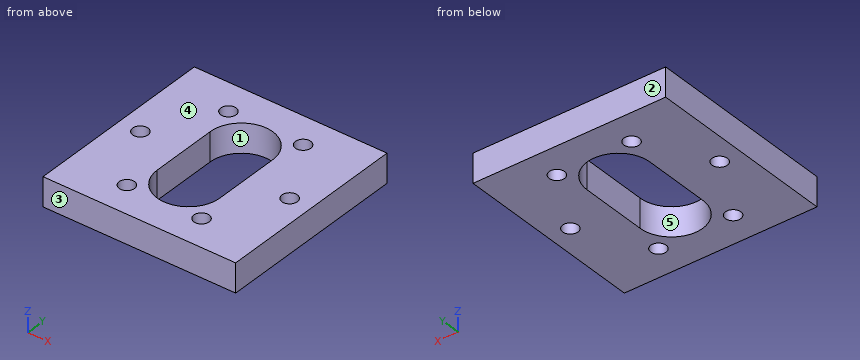
from build123d import *

# Parameters (mm, degrees)
SKETCH_1_W               = 40
SKETCH_1_H               = 40
EXTRUDE_1_DEPTH          = 6
CUT_EXTRUDE_1_DEPTH      = 29.91366459
CUT_EXTRUDE_1_DEPTH_BACK = 29.91366459
SKETCH_3_R               = 1.6
CUT_EXTRUDE_2_DEPTH      = 29.91366459


with BuildPart() as part:
    # 草圖1 → 填料-伸長1 (new body)
    with BuildSketch(Plane.XY):
        Rectangle(SKETCH_1_W, SKETCH_1_H)
    extrude(amount=EXTRUDE_1_DEPTH)

    # 草圖2 → 除料-伸長1 (cut, two sides: drawn at the far end of the back side and taken through both)
    with BuildSketch(Plane.XY.offset(6).offset(-CUT_EXTRUDE_1_DEPTH_BACK)):
        with BuildLine():
            Line((-6.5, -7), (-6.5, 7))
            ThreePointArc((-6.5, 7), (0, 13.5), (6.5, 7))
            Line((6.5, 7), (6.5, -7))
            ThreePointArc((6.5, -7), (0, -13.5), (-6.5, -7))
        make_face()
    extrude(amount=CUT_EXTRUDE_1_DEPTH + CUT_EXTRUDE_1_DEPTH_BACK, mode=Mode.SUBTRACT)

    # 草圖3 → 除料-伸長2 (cut, through all)
    with BuildSketch(Plane.XY.offset(6)):
        with Locations((-15.5, 0)):
            Circle(SKETCH_3_R)
        with Locations((-7.75, 13.423393759)):
            Circle(SKETCH_3_R)
        with Locations((7.75, 13.423393759)):
            Circle(SKETCH_3_R)
        with Locations((15.5, 0)):
            Circle(SKETCH_3_R)
        with Locations((7.75, -13.423393759)):
            Circle(SKETCH_3_R)
        with Locations((-7.75, -13.423393759)):
            Circle(SKETCH_3_R)
    extrude(amount=-CUT_EXTRUDE_2_DEPTH, mode=Mode.SUBTRACT)


solid = part.part
Design review of the part built by this model. Coordinates are the model's own, in mm. Face numbers are marked on the shaded views. A direction names the side the tool comes from. Coordinates: 2 decimals unless noted, no trailing zeros. Write each loop counter-clockwise with the first axis right and the second up, starting at its lowest first coordinate (ties: lowest second). Pieces come first, ordered by that corner, then holes. Notation, with made-up numbers: (64.5, 41.25) - (113.5, 41.25) arc R22 ccw to (113.5, 80.25) - close; hole circle Ø4 at (-18, 60.25). An arc over 180 degrees is marked (long way). One line per item, written item: value.
1) Add section D-D (y = 0). State the section outline as (x, z) points, plus the area to 3 significant figures.
Answer sheet:
outline: (-20, 0) - (-17.1, 0) - (-17.1, 6) - (-20, 6) - close; (-13.9, 0) - (-6.5, 0) - (-6.5, 6) - (-13.9, 6) - close; (6.5, 0) - (13.9, 0) - (13.9, 6) - (6.5, 6) - close; (17.1, 0) - (20, 0) - (20, 6) - (17.1, 6) - close
area: 124 mm2
2) Add section B-B (y = -4.5). State the section outline as (x, z) points, plus the area to 3 significant figures.
Answer sheet:
outline: (-20, 0) - (-6.5, 0) - (-6.5, 6) - (-20, 6) - close; (6.5, 0) - (20, 0) - (20, 6) - (6.5, 6) - close
area: 162 mm2
3) For the marked faces 1 and 2, list the 3-axis set-ups (+Z, -Z, +X, -X, +Y, -Y) from which the entire face can be reached by the end or side of a thin tool; tool diameter is ignored.
Answer sheet:
face 1: +Z, -Z
face 2: +Z, -Z, +X, -X, +Y
4) Add section C-C (x = 7.75). State the section outline as (y, z) points.
Answer sheet:
outline: (-20, 0) - (-15.02, 0) - (-15.02, 6) - (-20, 6) - close; (-11.82, 0) - (11.82, 0) - (11.82, 6) - (-11.82, 6) - close; (15.02, 0) - (20, 0) - (20, 6) - (15.02, 6) - close
5) Insertion check: pin 1 (2.5 mm diameter, centred on x = 7.75, y = -13.42, fed in from +Z). The pin has a flat end and moves straight along its axis. Give the tip position at first contact, or say it passes through.
Answer sheet:
pin 1: passes through
6) Mouldability with a two-part tool opening along Y and no side actions: class the marked faces 3, 4 and 5 as +Y half, -Y half, draft (parallel to the pull), parting line (faces both ways), or undercut.
Answer sheet:
face 3: -Y half
face 4: draft
face 5: undercut
7) Add section A-A (x = -15.5). State the section outline as (y, z) points.
Answer sheet:
outline: (-20, 0) - (-1.6, 0) - (-1.6, 6) - (-20, 6) - close; (1.6, 0) - (20, 0) - (20, 6) - (1.6, 6) - close
8) To check wall thickness, follow probe 1 along Y at (x, z) = (7.75, 1.85); probe 2 along X at (y, z) = (-2, 4.1); probe 3 along X at (y, z) = (1, 3). State the ranges of each line that lie inside material, in increasing order.
Answer sheet:
probe 1: y = -20 to -15.02, -11.82 to 11.82, 15.02 to 20
probe 2: x = -20 to -6.5, 6.5 to 20
probe 3: x = -20 to -16.75, -14.25 to -6.5, 6.5 to 14.25, 16.75 to 20
